Geometry: see drawing. Coordinates: mm, zero at the bounding-box minimum. Coordinates: 2 decimals unless noted, no trailing zeros. Order: outer loops, then holes, each group sorted by start corner. A loop starts at its lowest first (then second) coordinate and runs counter-clockwise, first axis right, second up. Notation, with made-up numbers: M -4.5,65.5 L 14.5,65.5 A21 ccw 14.5,80.5 Z; hole C 10,65.25 d5. An arc over 180 degrees is marked long. Answer in a Markdown table with one row per item.
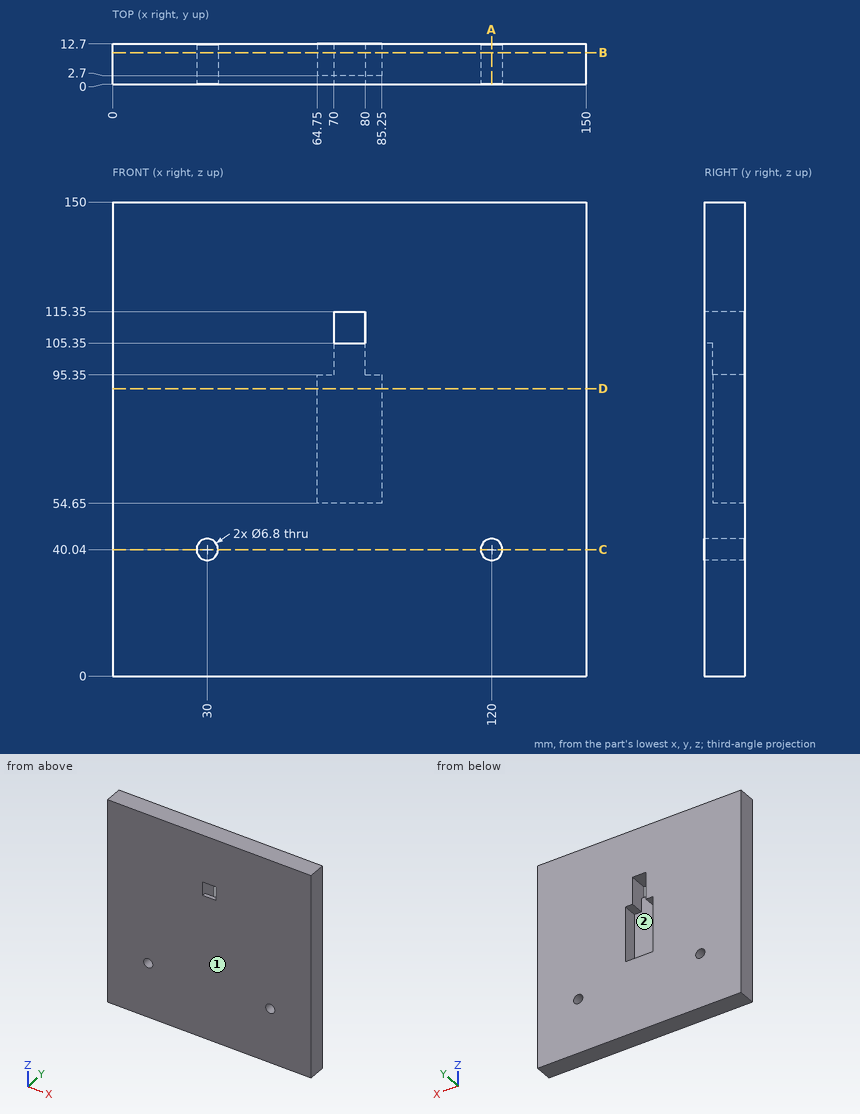
1) Material intervals for probe 1 along X at (y, z) = (3, 40.04); probe 2 along Z at (x, y) = (81, 4.5); probe 3 along X at (y, z) = (5.5, 76), sorted ascending.
Resolved:
| item | result |
|---|---|
| probe 1 | x = 0 to 26.6, 33.4 to 116.6, 123.4 to 150 |
| probe 2 | z = 0 to 54.65, 95.35 to 150 |
| probe 3 | x = 0 to 64.75, 85.25 to 150 |
2) Mould query, pull axis Z, two halves, no side actions, for the marked faces 1 and 2. Classes: +Z half, -Z half, draft (parallel to the pull), parting line (faces both ways), or undercut.
Resolved:
| item | result |
|---|---|
| face 1 | draft |
| face 2 | undercut |
3) Cut plane D-D, the plane z = 91. Output: boundary loops of the cut face in (x, y), and give its area (3 significant figures).
Resolved:
| item | result |
|---|---|
| outline | M 0,0 L 150,0 L 150,12.7 L 85.25,12.7 L 85.25,2.7 L 64.75,2.7 L 64.75,12.7 L 0,12.7 Z |
| area | 1,700 mm2 |
4) Cut plane C-C, the plane z = 40.04. Output: boundary loops of the cut face in (x, y).
Resolved:
| item | result |
|---|---|
| outline | M 0,0 L 26.6,0 L 26.6,12.7 L 0,12.7 Z; M 33.4,0 L 116.6,0 L 116.6,12.7 L 33.4,12.7 Z; M 123.4,0 L 150,0 L 150,12.7 L 123.4,12.7 Z |
5) Cut plane A-A, the plane x = 120. Output: boundary loops of the cut face in (y, z).
Resolved:
| item | result |
|---|---|
| outline | M 0,0 L 12.7,0 L 12.7,36.64 L 0,36.64 Z; M 0,43.44 L 12.7,43.44 L 12.7,150 L 0,150 Z |
6) Contact query for a flat-ended pin moving along its axis: pin 1 (6 mm diameter, centred on x = 71.5, z = 90.5, fed in from +Y). Output: stop coordinate, or through.
Resolved:
| item | result |
|---|---|
| pin 1 | stops at y = 2.7 |
7) Cut plane B-B, the plane y = 10. Output: boundary loops of the cut face in (x, z), and give its area (3 significant figures).
Resolved:
| item | result |
|---|---|
| outline | M 0,0 L 150,0 L 150,150 L 0,150 Z; hole C 30,40.04 d6.8; hole M 64.75,54.65 L 85.25,54.65 L 85.25,95.35 L 80,95.35 L 80,115.35 L 70,115.35 L 70,95.35 L 64.75,95.35 Z; hole C 120,40.04 d6.8 |
| area | 21,400 mm2 |
